```python
from build123d import *

# Parameters (mm, degrees)
F2_DEPTH = 30
F3_W     = 630
F3_H     = 18
F4_DEPTH = 600
F5_W     = 264.534249
F5_H     = 18
F6_DEPTH = 500


with BuildPart() as f2:
    # F1 (on offset) → F2 (new body)
    with BuildSketch(Plane.YZ.offset(500)):
        Polygon((-543.262288, 0), (-331.96829, 393.950819), (-267.480748, 0), (0, 0), (-182.519252, 1115), (-450, 1115), (-345.235586, 475), (-600, 0), align=None)
        Polygon((-225, 50), (-391.149812, 1065), (-225, 1065), (-58.850188, 50), align=None, mode=Mode.SUBTRACT)
    extrude(amount=F2_DEPTH)

    # F3 (on Front) → F4 (join)
    with BuildSketch(Plane.XZ):
        with Locations((315, 1124)):
            Rectangle(F3_W, F3_H)
    extrude(amount=F4_DEPTH)

    # F5 (on Right) → F6 (join, through all)
    with BuildSketch(Plane.YZ):
        with Locations((-282.047497, 906)):
            Rectangle(F5_W, F5_H)
        with Locations((-233.430262, 609)):
            Rectangle(F5_W, F5_H)
        with Locations((-167.952503, 209)):
            Rectangle(F5_W, F5_H)
    extrude(amount=F6_DEPTH)

    # F7: F2 across plane


with BuildPart() as f2_1:
    add(f2.part)
    add(f2.part.mirror(Plane.YZ))


solid = f2_1.part
```
For this review, take the finished solid that the model builds, in its own axes (mm). A direction names the side the tool comes from. Round coordinates to 2 decimals unless told otherwise and drop trailing zeros. Write each loop counter-clockwise with the first axis right and the second up, starting at its lowest first coordinate (ties: lowest second). Pieces come first, ordered by that corner, then holes. Notation, with made-up numbers: (-3.5, -6.75) - (9.5, -6.75) arc R29 ccw to (9.5, 21.25) - close; hole circle Ø5 at (-10, 68.25). An arc over 180 degrees is marked (long way). Answer as a JSON object with one key per item and string values.
1. We need section A-A on x = 288. Give the boundary of the cut face in (y, z), then the cut area to 3 significant figures.
Response values:
{"outline": "(-600, 1115) - (0, 1115) - (0, 1133) - (-600, 1133) - close; (-414.31, 897) - (-149.78, 897) - (-149.78, 915) - (-414.31, 915) - close; (-365.7, 600) - (-101.16, 600) - (-101.16, 618) - (-365.7, 618) - close; (-300.22, 200) - (-35.69, 200) - (-35.69, 218) - (-300.22, 218) - close", "area": "25,100 mm2"}
2. We need section B-B on z = 103. Give the boundary of the cut face in (x, y).
Response values:
{"outline": "(-530, -544.76) - (-500, -544.76) - (-500, -488.02) - (-530, -488.02) - close; (-530, -284.34) - (-500, -284.34) - (-500, -233.68) - (-530, -233.68) - close; (-530, -67.53) - (-500, -67.53) - (-500, -16.86) - (-530, -16.86) - close; (500, -544.76) - (530, -544.76) - (530, -488.02) - (500, -488.02) - close; (500, -284.34) - (530, -284.34) - (530, -233.68) - (500, -233.68) - close; (500, -67.53) - (530, -67.53) - (530, -16.86) - (500, -16.86) - close"}
3. We need section C-C on z = 878. Give the boundary of the cut face in (x, y), then the cut area to 3 significant figures.
Response values:
{"outline": "(-530, -411.2) - (-500, -411.2) - (-500, -360.54) - (-530, -360.54) - close; (-530, -194.39) - (-500, -194.39) - (-500, -143.72) - (-530, -143.72) - close; (500, -411.2) - (530, -411.2) - (530, -360.54) - (500, -360.54) - close; (500, -194.39) - (530, -194.39) - (530, -143.72) - (500, -143.72) - close", "area": "6,080 mm2"}
4. Draft analysis for pull direction X (two halves, no side actions). For faces 1 (the face through (514.79, -470.834, 240.825)), 2 (the face through (-530, -301, 478)), 3 (the face through (500, -302, 1080)), state which applies: +X half, -X half, draft (parallel to the pull), parting line (faces both ways), or undercut.
Response values:
{"face 1": "draft", "face 2": "-X half", "face 3": "undercut"}
5. To check wall thickness, follow line 1 along Z through (x, y) = (-485, -349); line 2 along Z through (x, y) = (-483, -182.5); line 3 along Z through (x, y) = (127.5, -125). State the ranges of each line that lie inside material, in increasing order.
Response values:
{"line 1": "z = 600 to 618, 897 to 915, 1115 to 1133", "line 2": "z = 200 to 218, 600 to 618, 897 to 915, 1115 to 1133", "line 3": "z = 200 to 218, 600 to 618, 1115 to 1133"}
6. Tool access review of faces 4 (the face through (514.79, -89.982, 549.695)), 5 (the face through (7, -235, 618)), 6 (the face through (-514.79, -470.834, 240.825)): name each direction out of +Z, -Z, +X, -X, +Y, -Y from which nothing blocks a thin tool from reaching the whole face with its end or side.
Response values:
{"face 4": "+X, -X, +Y", "face 5": "+Y, -Y", "face 6": "+X, -X, -Y"}
7. For pin 1 Ø5.5 at (x, z) = (-200, 605.5) entering from +Y; pin 2 Ø4 at (x, y) = (-52, -235.5) entering from -Z; pin 3 Ø14.5 at (y, z) = (-139, 207.5) entering from +X, all flat-tipped, find the tip position at first contact; note any pin that passes through.
Response values:
{"pin 1": "stops at y = -101.16", "pin 2": "stops at z = 200", "pin 3": "stops at x = 500"}
